Build history of the part. All positions in model axes, mm. A direction names the side the tool comes from. Round coordinates to 2 decimals unless told otherwise and drop trailing zeros. Order: outer loops, then holes, each group sorted by start corner. A loop starts at its lowest first (then second) coordinate and runs counter-clockwise, first axis right, second up. Notation, with made-up numbers: (75, -23.5) -> (99, -23.5) arc R23 cw to (99, -4.5) -> close; hole circle Ø9 at (86, 64). An arc over 180 degrees is marked (long way). Answer as a JSON object with one key per item and string values.
from build123d import *

# Parameters (mm, degrees)
SKETCH_1_R          = 7.5
SKETCH_1_R_2        = 5
SKETCH_1_W          = 4
SKETCH_1_H          = 25
EXTRUDE_1_DEPTH     = 40
SKETCH_3_R          = 5
EXTRUDE_2_DEPTH     = 3
SKETCH_4_R          = 3
CUT_EXTRUDE_2_DEPTH = 54.867163989


with BuildPart() as part:
    # Эскиз1 → Бобышка-Вытянуть1 (new body)
    # profile 1 of 3: a face of its own
    with BuildSketch(Plane.XY):
        Circle(SKETCH_1_R)
        Circle(SKETCH_1_R_2, mode=Mode.SUBTRACT)
    # profile 2 of 3: a face of its own
    with BuildSketch(Plane.XY):
        with Locations((0, 35)):
            Circle(SKETCH_1_R)
        with Locations((0, 35)):
            Circle(SKETCH_1_R_2, mode=Mode.SUBTRACT)
    # profile 3 of 3: a face of its own
    with BuildSketch(Plane.XY):
        with Locations((0, 17.5)):
            Rectangle(SKETCH_1_W, SKETCH_1_H)
    extrude(amount=EXTRUDE_1_DEPTH)

    # Эскиз3 → Бобышка-Вытянуть2 (add, symmetric)
    with BuildSketch(Plane(origin=(0, 0, 10), x_dir=(-1, 0, 0), z_dir=(0, 0, -1))):
        with BuildLine():
            Line((-5.924618308, 4.598793093), (-18.091881162, -11.076273562))
            ThreePointArc((-18.091881162, -11.076273562), (-12.52175414, -9.411980886), (-9.142135624, -14.142135624))
            ThreePointArc((-9.142135624, -14.142135624), (-9.651628397, -16.34107738), (-11.076273562, -18.091881162))
            Line((-11.076273562, -18.091881162), (4.598793093, -5.924618308))
            Line((4.598793093, -5.924618308), (3.065862062, -3.949745538))
            ThreePointArc((3.065862062, -3.949745538), (-3.535533906, -3.535533906), (-3.949745538, 3.065862062))
            Line((-3.949745538, 3.065862062), (-5.924618308, 4.598793093))
        make_face()
        with Locations((-14.142135624, -14.142135624)):
            Circle(SKETCH_3_R)
    extrude(amount=EXTRUDE_2_DEPTH, both=True)

    # Эскиз4 → Вырез-Вытянуть2 (cut, through all)
    with BuildSketch(Plane.XY.offset(13)):
        with Locations((14.142135624, -14.142135624)):
            Circle(SKETCH_4_R)
    extrude(amount=-CUT_EXTRUDE_2_DEPTH, mode=Mode.SUBTRACT)


solid = part.part
1) Cut at A-A, the plane y = 35. Give the cut face in (x, z), plus the area to 3 significant figures.
Checked values:
{"outline": "(-7.5, 0) -> (-5, 0) -> (-5, 40) -> (-7.5, 40) -> close; (5, 0) -> (7.5, 0) -> (7.5, 40) -> (5, 40) -> close", "area": "200 mm²"}
2) Probe L1, parallel to Y at x = 0, z = 16; L2, parallel to X at y = 35, z = 22; L3, parallel to Y at x = 0, z = 9.5. List the from-to ranges inside material, lowest first. Write a range as from..to.
Checked values:
{"L1": "y = -7.5..-5, 5..30, 40..42.5", "L2": "x = -7.5..-5, 5..7.5", "L3": "y = -9.49..-5, 5..30, 40..42.5"}
3) Cut at D-D, the plane z = 34. Give the cut face in (x, y), plus the area to 3 significant figures.
Checked values:
{"outline": "(-2, 7.23) arc R7.5 ccw (long way) to (2, 7.23) -> (2, 27.77) arc R7.5 ccw (long way) to (-2, 27.77) -> close; hole circle Ø10 at (0, 0); hole circle Ø10 at (0, 35)", "area": "277 mm²"}
4) Cut at C-C, the plane x = 1.25. Give the cut face in (y, z), plus the area to 3 significant figures.
Checked values:
{"outline": "(-10.46, 7) -> (-7.4, 7) -> (-7.4, 0) -> (-4.84, 0) -> (-4.84, 40) -> (-7.4, 40) -> (-7.4, 13) -> (-10.46, 13) -> close; (4.84, 0) -> (30.16, 0) -> (30.16, 40) -> (4.84, 40) -> close; (39.84, 0) -> (42.4, 0) -> (42.4, 40) -> (39.84, 40) -> close", "area": "1,240 mm²"}
5) Which spindle directions (+Z, -Z, +X, -X, +Y, -Y) get a long thin tool onto all of the face, cutting with end or side? Do faces 1 (the face through (2, 17, 20)), 2 (the face through (3.348, -12.093, 9.958)), 3 (the face through (-2, 17, 20)). Say none if no direction does.
Checked values:
{"face 1": "+Z, -Z, +X", "face 2": "+Z, -Z, -X, -Y", "face 3": "+Z, -Z, -X"}
6) Pull direction X, two halves, no side cores. Call faces 4 (the face through (-4.706, -5.84, 19.72)), 5 (the face through (15.75, -11.61, 10.04)), 6 (the face through (0, 18, 40)): pulls with the +X half, pulls with the -X half, needs draft (parallel to the pull), parting line crosses it, or undercut.
Checked values:
{"face 4": "parting line crosses it", "face 5": "undercut", "face 6": "needs draft"}
7) Cut at B-B, the plane x = 15.25. Give the cut face in (y, z), plus the area to 3 significant figures.
Checked values:
{"outline": "(-19.02, 7) -> (-16.93, 7) -> (-16.93, 13) -> (-19.02, 13) -> close; (-11.35, 7) -> (-7.42, 7) -> (-7.42, 13) -> (-11.35, 13) -> close", "area": "36.2 mm²"}
8) Flat gauge pins, fed straight in: pin 1 Ø10 at (y, z) = (25, 12.5) entering from +X; pin 2 Ø6 at (y, z) = (-8, 28) entering from -X; pin 3 Ø1 at (x, z) = (1.5, 16) entering from +Y. Where does each tip first touch, or does it go through?
Checked values:
{"pin 1": "stops at x = 5.59", "pin 2": "stops at x = -5.59", "pin 3": "stops at y = 42.43"}
